from build123d import *

# Parameters (mm, degrees)
CORTAR_EXTRUIR1_DEPTH = 2
CHAFL_N1_SIZE         = 0.5
REDONDEO1_R           = 0.5


with BuildPart() as part:
    # Croquis1 → Revolución1 (revolve)
    with BuildSketch(Plane.XY):
        Polygon((0, 0), (2.75, 0), (2.75, -3), (1.5, -3), (1.5, -13), (0, -13), align=None)
    revolve(axis=Axis((0, 0, 0), (0, -1, 0)))

    # Croquis2 → Cortar-Extruir1 (cut)
    with BuildSketch(Plane(origin=(0, 0, 0), x_dir=(1, 0, 0), z_dir=(0, 1, 0))):
        Polygon((1.25, 0.721687836), (0, 1.443375673), (-1.25, 0.721687836), (-1.25, -0.721687836), (0, -1.443375673), (1.25, -0.721687836), align=None)
    extrude(amount=-CORTAR_EXTRUIR1_DEPTH, mode=Mode.SUBTRACT)

    # Chaflán1
    chafl_n1_edges = [part.edges().sort_by_distance(p)[0] for p in [
        (-1.5, -13, 0),
    ]]
    chamfer(chafl_n1_edges, length=CHAFL_N1_SIZE)

    # Redondeo1
    redondeo1_edges = [part.edges().sort_by_distance(p)[0] for p in [
        (-2.75, 0, 0),
    ]]
    fillet(redondeo1_edges, radius=REDONDEO1_R)


solid = part.part
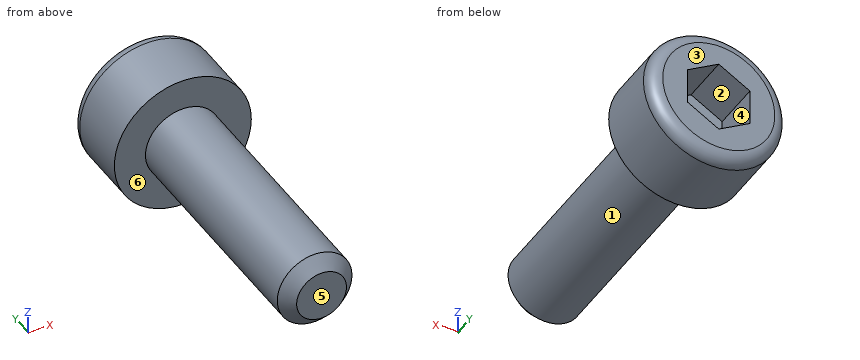
Source: CAD feature listing. Evaluate the final solid. Frame: model axes, mm. Face numbers are marked on the shaded views. A direction names the side the tool comes from. Round coordinates to 2 decimals unless told otherwise and drop trailing zeros. Loops run counter-clockwise (first coordinate to the right, second up) from the corner with the lowest first, then second, coordinate; pieces in that order, holes last.
Q1. Section A-A, the plane y = -1.25. Return loops of the section in (x, z).
Q2. First-contact query: P1, Ø1, axis at y = -11, z = 1.5, coming from the +X side; P2, Ø2, axis at y = -10.5, z = 1, coming from the +X side; P3, Ø0.8, axis at x = -0.5, z = -0.5, coming from the +Y side; P4, Ø3, axis at x = -1, z = -2, coming from the -Y side. Flat tips, straight axial feed; report the tip coordinate or a pass-through.
Q3. Access query for the marked faces 4, 5 and 6. Directions: +Z, -Z, +X, -X, +Y, -Y. A direction counts if a zero-diameter tool reaches every point of the face in a straight line with its end or side. Return the directions, or none.
Q4. Section B-B, the plane z = 0. Return loops of the section in (x, y).
Q5. Ray query, line 1 (Z direction, x = 0, y = -7.75); line 2 (X direction, y = -1.5, z = -2.45). Return the intervals inside material, ascending.
Q6. Mould query, pull axis X, two halves, no side actions, for the marked faces 1, 2 and 3. Classes: pulls with the +X half, pulls with the -X half, needs draft (parallel to the pull), parting line crosses it, or undercut.
Q7. Section C-C, the plane y = -3.5. Return loops of the section in (x, z), plus the area to 3 significant figures.
Solutions:
1. outline: circle Ø5.5 at (0, 0); hole (-1.25, -0.72) - (0, -1.44) - (1.25, -0.72) - (1.25, 0.72) - (0, 1.44) - (-1.25, 0.72) - close
2. P1: stops at x = 1.12
2. P2: stops at x = 1.5
2. P3: stops at y = -2
2. P4: stops at y = -13
3. face 4: +Y
3. face 5: +Z, -Z, +X, -X, -Y
3. face 6: -Y
4. outline: (-2.75, -3) - (-1.5, -3) - (-1.5, -12.5) - (-1, -13) - (1, -13) - (1.5, -12.5) - (1.5, -3) - (2.75, -3) - (2.75, -0.5) arc R0.5 ccw to (2.25, 0) - (1.25, 0) - (1.25, -2) - (-1.25, -2) - (-1.25, 0) - (-2.25, 0) arc R0.5 ccw to (-2.75, -0.5) - close
5. line 1: z = -1.5 to 1.5
5. line 2: x = -1.25 to 1.25
6. face 1: parting line crosses it
6. face 2: undercut
6. face 3: needs draft
7. outline: circle Ø3 at (0, 0)
7. area: 7.07 mm2
